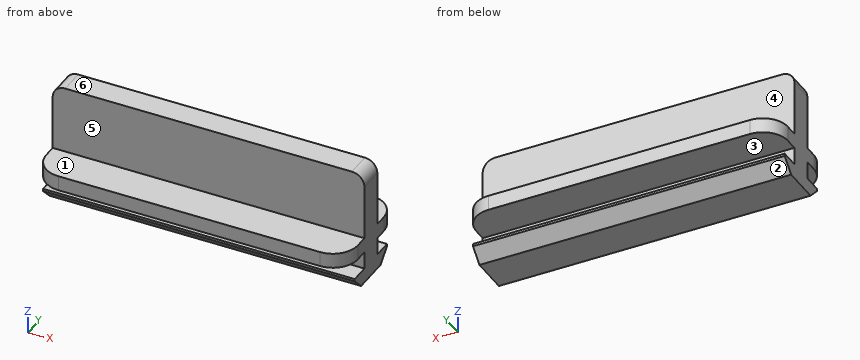
Autodesk Inventor part; units mm, degrees
ref_plane "YZ Plane" through (0, 0, 0) normal (1, 0, 0) x (0, 1, 0)
ref_plane "XZ Plane" through (0, 0, 0) normal (0, 1, 0) x (-1, 0, 0)
ref_plane "XY Plane" through (0, 0, 0) normal (0, 0, 1) x (1, 0, 0)
sketch "Sketch1" plane through (0, 0, 0) normal (0, 0, 1) x (1, 0, 0)
  line L0 (-9.2369, 2.8715) -> (15.6631, 2.8715)
  line L1 (15.6631, 2.8715) -> (15.6631, -2.1285)
  line L2 (15.6631, -2.1285) -> (-9.2369, -2.1285)
  line L3 (-9.2369, -2.1285) -> (-9.2369, 2.8715)
  point P0 (0, 0)
  dimension "d0" = 24.9
  dimension "d1" = 5
extrude "Extrusion1" add sketch "Sketch1" along normal blind 1.2
sketch "Sketch2" plane through (0, 0, 1.2) normal (0, 0, 1) x (1, 0, 0)
  line L0 (-9.2369, 2.8715) -> (-9.2369, -2.1285)
  line L1 (15.6631, -2.1285) -> (15.6631, 2.8715)
  line L2 (-9.2369, 1.3715) -> (15.6631, 1.3715)
  line L3 (15.6631, 1.3715) -> (15.6631, -0.6285)
  line L4 (15.6631, -0.6285) -> (-9.2369, -0.6285)
  line L5 (-9.2369, -0.6285) -> (-9.2369, 1.3715)
  line L6 (15.6631, 2.8715) -> (-9.2369, 2.8715)
  point P0 (0, 0)
  point P1 (15.6631, 1.3715)
  dimension "d4" = 2
  dimension "d5" = 1.5
extrude "Extrusion2" add sketch "Sketch2" along normal blind 8 contours L2 L1 L4 L0
chamfer "Chamfer1" distance 1 angle 45 2 edges at (3.2131, 2.8715, 0) (3.2131, -2.1285, 0)
fillet "Fillet4" radius 1 2 edges at (-9.2369, 0.3715, 9.2) (15.6631, 0.3715, 9.2)
sketch "Sketch3" plane through (-9.2369, 1.3715, 1.2) normal (0, 1, 0) x (1, 0, 0)
  line L0 (0, 0) -> (0, -7)
  line L1 (24.9, 0) -> (24.9, -7)
  line L2 (0, -1.4) -> (24.9, -1.4)
  line L3 (24.9, -1.4) -> (24.9, -2.6)
  line L4 (24.9, -2.6) -> (0, -2.6)
  line L5 (0, -2.6) -> (0, -1.4)
  line L6 (24.9, 0) -> (0, 0)
  point P0 (9.2369, 1.2)
  point P1 (0, -2.6)
  dimension "d15" = 1.4
  dimension "d16" = 1.2
extrude "Extrusion3" add sketch "Sketch3" along normal blind 3 contours L2 L1 L4 L0
sketch "Sketch4" plane through (-9.2369, -0.6285, 1.2) normal (0, -1, 0) x (1, 0, 0)
  line L0 (24.9, 2.6) -> (0, 2.6)
  line L1 (0, 1.4) -> (24.9, 1.4)
  line L2 (24.9, 2.6) -> (0, 2.6)
  line L3 (0, 2.6) -> (0, 1.4)
  line L4 (0, 1.4) -> (24.9, 1.4)
  line L5 (24.9, 1.4) -> (24.9, 2.6)
  point P0 (9.2369, -1.2)
  point P1 (0, 2.6)
extrude "Extrusion4" add sketch "Sketch4" along normal blind 3
fillet "Fillet5" radius 2 4 edges at (-9.2369, 4.3715, 3.2) (-9.2369, -3.6285, 3.2) (15.6631, 4.3715, 3.2) (15.6631, -3.6285, 3.2)
properties part number "flag"
CAD build for the part. Positions are in the model's coordinates, mm. Face numbers are marked on the shaded views. A direction names the side the tool comes from. Give positions to 0.01 mm unless a question says otherwise; leave off trailing zeros. Write each loop counter-clockwise with the first axis right and the second up, starting at its lowest first coordinate (ties: lowest second). Pieces come first, ordered by that corner, then holes. Notation, with made-up numbers: M 14,8.5 L 62,8.5 A23 ccw 62,36.5 Z; hole C 5.5,-15 d11. An arc over 180 degrees is marked long. Put each result on its own line as item: value. Start each with the question number.
(1) Probe L1, parallel to Z at x = -5.25, y = 1.5; L2, parallel to Z at x = -7.5, y = 3; L3, parallel to Y at x = -7.25, z = 7. List the from-to ranges inside material, lowest first.
(2) Band-saw the part on C-C, the plane y = -2.75. Write the cut outline in (x, z).
(3) Band-saw the part on B-B, the plane x = 11.25. Write the cut outline in (y, z).
(4) Flat gauge pins, fed straight in: pin 1 Ø2.5 at (x, z) = (-2.5, 8) entering from -Y; pin 2 Ø1.5 at (x, y) = (8, -2.5) entering from +Z; pin 3 Ø0.7 at (x, z) = (6.5, 2) entering from +Y. Where does each tip first touch, or does it go through?
(5) Band-saw the part on A-A, the plane z = 3.25. Write the cut outline in (x, y), and give its area (3 significant figures).
(6) Mould opens along Z. For the marked faces 1, 2 and 3 say: +Z half, -Z half, draft (parallel to the pull), parting line (faces both ways), or undercut.
(7) Band-saw the part on D-D, the plane z = 5.5. Write the cut outline in (x, y).
(8) Which spindle directions (+Z, -Z, +X, -X, +Y, -Y) get a long thin tool onto all of the face, cutting with end or side? Do the marked faces 4, 5 and 6. Say none if no direction does.
Response values:
1. L1: z = 0 to 1.2, 2.6 to 3.8
1. L2: z = 2.6 to 3.8
1. L3: y = -0.63 to 1.37
2. outline: M -8.89,2.6 L 15.32,2.6 L 15.32,3.8 L -8.89,3.8 Z
3. outline: M -3.63,2.6 L -0.63,2.6 L -0.63,1.2 L -2.13,1.2 L -2.13,1 L -1.13,0 L 1.87,0 L 2.87,1 L 2.87,1.2 L 1.37,1.2 L 1.37,2.6 L 4.37,2.6 L 4.37,3.8 L 1.37,3.8 L 1.37,9.2 L -0.63,9.2 L -0.63,3.8 L -3.63,3.8 Z
4. pin 1: stops at y = -0.63
4. pin 2: stops at z = 3.8
4. pin 3: stops at y = 1.37
5. outline: M -9.24,-1.63 A2 ccw -7.24,-3.63 L 13.66,-3.63 A2 ccw 15.66,-1.63 L 15.66,2.37 A2 ccw 13.66,4.37 L -7.24,4.37 A2 ccw -9.24,2.37 Z
5. area: 196 mm2
6. face 1: +Z half
6. face 2: -Z half
6. face 3: undercut
7. outline: M -9.24,-0.63 L 15.66,-0.63 L 15.66,1.37 L -9.24,1.37 Z
8. face 4: +Z, +X, -X, +Y
8. face 5: +Z, +X, -X, -Y
8. face 6: +Z, +X, -X, +Y, -Y
